The listing builds one solid part. Answer for the finished solid, in the listing's coordinates (mm). Coordinates: 2 decimals unless noted, no trailing zeros. Order: outer loops, then holes, each group sorted by start corner. A loop starts at its lowest first (then second) coordinate and runs counter-clockwise, first axis right, second up.
from build123d import *

# Parameters (mm, degrees)
F0_R     = 11.2
F1_DEPTH = 5


with BuildPart() as f1:
    # F0 (on Top) → F1 (new body)
    with BuildSketch(Plane.XY):
        Polygon((49.999069, 0.305094), (24.735316, 43.453011), (-25.263753, 43.147917), (-49.999069, -0.305094), (-24.735316, -43.453011), (25.263753, -43.147917), align=None)
        with Locations((-16.835953, -29.011287)):
            Circle(F0_R, mode=Mode.SUBTRACT)
        with Locations((16.706536, -29.086007)):
            Circle(F0_R, mode=Mode.SUBTRACT)
        with Locations((33.542488, -0.074719)):
            Circle(F0_R, mode=Mode.SUBTRACT)
        with Locations((-33.542488, 0.074719)):
            Circle(F0_R, mode=Mode.SUBTRACT)
        with Locations((-16.706536, 29.086007)):
            Circle(F0_R, mode=Mode.SUBTRACT)
        Circle(F0_R, mode=Mode.SUBTRACT)
        with Locations((16.835953, 29.011287)):
            Circle(F0_R, mode=Mode.SUBTRACT)
    extrude(amount=F1_DEPTH)


solid = f1.part
1) Each of these flat-tipped pins is pushed along its axis until it touches: P1, Ø5, axis at x = -26, y = 31.5, coming from the +Z side; P2, Ø2, axis at y = 11, z = 3, coming from the -X side; P3, Ø1, axis at y = 14.5, z = 3, coming from the +X side; P4, Ø1, axis at y = -22, z = 2, coming from the +X side. Where does it stop, or does it pass through?
2) Consider L1, parallel to X at y = -5.5, z = 1.85; L2, parallel to Y at x = 24.5, z = 1.15; L3, parallel to X at y = 26.5, z = 1.15. Determine where each line is inside the solid, lowest interval first.
3) Section B-B (y = -27) is taken. Give the vertices of the cut face in (x, z), then the cut area to 3 significant figures.
4) Section D-D (z = 2.8) is taken. Give the vertices of the cut face in (x, y).
5) Determine the mould class of faces 1 (the face through (-37.458, 21.726, 2.465)), 2 (the face through (22.004, 19.075, 2.465)), 3 (the face through (10, 10, 0)) for opening direction Y: released by +Y, released by -Y, zero draft, split by the parting line, or undercut.
6) Section C-C (x = -7) is taken. Give the vertices of the cut face in (y, z), then the cut area to 3 significant figures.
7) Section A-A (x = -38.5) is taken. Give the vertices of the cut face in (y, z).
Filled sheet:
1. P1: stops at z = 5
1. P2: stops at x = -44.13
1. P3: stops at x = 41.98
1. P4: stops at x = 37.59
2. L1: x = -46.96 to -43.26, -23.83 to -9.76, 9.76 to 23.74, 43.34 to 46.69
2. L2: y = -43.15 to -37.13, -21.04 to -6.68, 6.53 to 20.84, 37.18 to 43.45
2. L3: x = -34.74 to -27.6, -5.81 to 5.92, 27.75 to 34.66
3. outline: (-34.37, 0) - (-27.85, 0) - (-27.85, 5) - (-34.37, 5) - close; (-5.82, 0) - (5.7, 0) - (5.7, 5) - (-5.82, 5) - close; (27.71, 0) - (34.46, 0) - (34.46, 5) - (27.71, 5) - close
3. area: 124 mm2
4. outline: (-50, -0.31) - (-24.74, -43.45) - (25.26, -43.15) - (50, 0.31) - (24.74, 43.45) - (-25.26, 43.15) - close; hole circle Ø22.4 at (-33.54, 0.07); hole circle Ø22.4 at (-16.84, -29.01); hole circle Ø22.4 at (-16.71, 29.09); hole circle Ø22.4 at (0, 0); hole circle Ø22.4 at (16.71, -29.09); hole circle Ø22.4 at (16.84, 29.01); hole circle Ø22.4 at (33.54, -0.07)
5. face 1: released by +Y
5. face 2: undercut
5. face 3: zero draft
6. outline: (-43.34, 0) - (-34.37, 0) - (-34.37, 5) - (-43.34, 5) - close; (-23.65, 0) - (-8.74, 0) - (-8.74, 5) - (-23.65, 5) - close; (8.74, 0) - (23.5, 0) - (23.5, 5) - (8.74, 5) - close; (34.67, 0) - (43.26, 0) - (43.26, 5) - (34.67, 5) - close
6. area: 236 mm2
7. outline: (-19.94, 0) - (-9.97, 0) - (-9.97, 5) - (-19.94, 5) - close; (10.12, 0) - (19.9, 0) - (19.9, 5) - (10.12, 5) - close
